CAD build for the part. Positions are in the model's coordinates, mm. Face numbers are marked on the shaded views. A direction names the side the tool comes from. Coordinates: 2 decimals unless noted, no trailing zeros. Loops run counter-clockwise (first coordinate to the right, second up) from the corner with the lowest first, then second, coordinate; pieces in that order, holes last. Notation, with made-up numbers: (-21.75, 6.25) - (19.25, 6.25) arc R11 ccw to (19.25, 16.25) - close; hole circle Ø1 at (-16.75, -28.75). An arc over 180 degrees is marked (long way). Put each result on its own line as item: value.
```python
from build123d import *

# Parameters (mm, degrees)
SCHIZZO1_W                        = 27
SCHIZZO1_H                        = 36
ESTRUSIONE_ESTRUSIONE1_DEPTH      = 4
SCHIZZO10_R                       = 1.75
TAGLIO_ESTRUSIONE5_DEPTH          = 10
SCHIZZO12_W                       = 124
SCHIZZO12_H                       = 2.549259356
ESTRUSIONE_ESTRUSIONE2_DEPTH      = 55
ESTRUSIONE_ESTRUSIONE2_DEPTH_BACK = 55
SCHIZZO14_W                       = 3
SCHIZZO14_H                       = 1.5
ESTRUSIONE_ESTRUSIONE3_DEPTH      = 110
SCHIZZO15_W                       = 27
SCHIZZO15_H                       = 4
TAGLIO_ESTRUSIONE6_DEPTH          = 5
SCHIZZO16_R                       = 13.5
TAGLIO_ESTRUSIONE7_DEPTH          = 10


with BuildPart() as part:
    # Schizzo1 → Estrusione-Estrusione1 (new body)
    with BuildSketch(Plane.XY):
        with Locations((13.5, -18)):
            Rectangle(SCHIZZO1_W, SCHIZZO1_H)
    extrude(amount=ESTRUSIONE_ESTRUSIONE1_DEPTH)

    # Schizzo10 → Taglio-Estrusione5 (cut)
    with BuildSketch(Plane.XY.offset(4)):
        with Locations((3.5, -12.5)):
            Circle(SCHIZZO10_R)
        with Locations((23.5, -12.5)):
            Circle(SCHIZZO10_R)
        with Locations((23.5, -27.5)):
            Circle(SCHIZZO10_R)
        with Locations((3.5, -27.5)):
            Circle(SCHIZZO10_R)
    extrude(amount=-TAGLIO_ESTRUSIONE5_DEPTH, mode=Mode.SUBTRACT)

    # Schizzo12 → Estrusione-Estrusione2 (add, two sides)
    with BuildSketch(Plane(origin=(13.5, 0, 0), x_dir=(0, 0, -1), z_dir=(1, 0, 0))) as estrusione_estrusione2_sk:
        with Locations((-66, -34.725370322)):
            Rectangle(SCHIZZO12_W, SCHIZZO12_H)
    extrude(amount=ESTRUSIONE_ESTRUSIONE2_DEPTH)
    extrude(estrusione_estrusione2_sk.sketch, amount=-ESTRUSIONE_ESTRUSIONE2_DEPTH_BACK)

    # Schizzo14 → Estrusione-Estrusione3 (add)
    with BuildSketch(Plane.ZY.offset(41.5)):
        with Locations((104, -32.700740644)):
            Rectangle(SCHIZZO14_W, SCHIZZO14_H)
        with Locations((119, -32.700740644)):
            Rectangle(SCHIZZO14_W, SCHIZZO14_H)
    extrude(amount=-ESTRUSIONE_ESTRUSIONE3_DEPTH)

    # Schizzo15 → Taglio-Estrusione6 (cut, through all)
    with BuildSketch(Plane.XY.offset(4)):
        with Locations((13.5, -2)):
            Rectangle(SCHIZZO15_W, SCHIZZO15_H)
    extrude(amount=-TAGLIO_ESTRUSIONE6_DEPTH, mode=Mode.SUBTRACT)

    # Schizzo16 → Taglio-Estrusione7 (cut)
    with BuildSketch(Plane(origin=(0, -33.450740644, 0), x_dir=(1, 0, 0), z_dir=(0, 1, 0))):
        with Locations((29.5, -45)):
            Circle(SCHIZZO16_R)
    extrude(amount=-TAGLIO_ESTRUSIONE7_DEPTH, mode=Mode.SUBTRACT)


solid = part.part
```
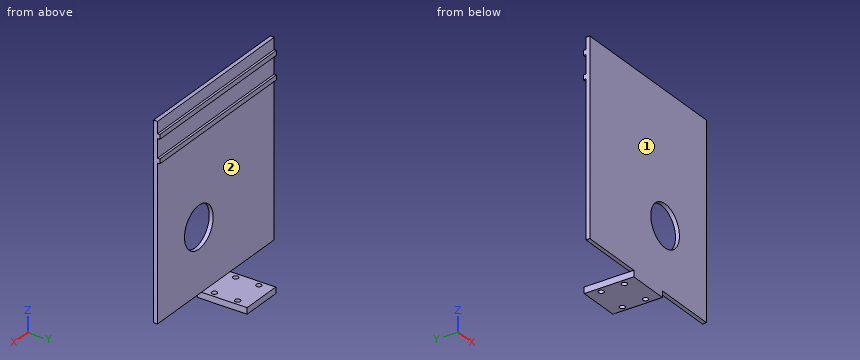
Q1. Slice it at A-A, the plane x = 3.5. Give the cut face in (y, z), then the cut area to 3 significant figures.
Determined:
outline: (-36, 0) - (-29.25, 0) - (-29.25, 4) - (-33.45, 4) - (-33.45, 102.5) - (-31.95, 102.5) - (-31.95, 105.5) - (-33.45, 105.5) - (-33.45, 117.5) - (-31.95, 117.5) - (-31.95, 120.5) - (-33.45, 120.5) - (-33.45, 128) - (-36, 128) - close; (-25.75, 0) - (-14.25, 0) - (-14.25, 4) - (-25.75, 4) - close; (-10.75, 0) - (-4, 0) - (-4, 4) - (-10.75, 4) - close
area: 425 mm2
Q2. Wall check: L1, parallel to Y at x = 23.5, z = 1.2; L2, parallel to X at y = -34.1, z = 45; L3, parallel to Z at x = 29.5, y = -34.95. Give the ranges that are in metal, low to high. Write a range as from..to.
Determined:
L1: -36..-29.25, -25.75..-14.25, -10.75..-4
L2: -41.5..16, 43..68.5
L3: 4..31.5, 58.5..128
Q3. Slice it at D-D, the plane x = 29.5. Give the cut face in (y, z), then the cut area to 3 significant figures.
Determined:
outline: (-36, 4) - (-33.45, 4) - (-33.45, 31.5) - (-36, 31.5) - close; (-36, 58.5) - (-33.45, 58.5) - (-33.45, 102.5) - (-31.95, 102.5) - (-31.95, 105.5) - (-33.45, 105.5) - (-33.45, 117.5) - (-31.95, 117.5) - (-31.95, 120.5) - (-33.45, 120.5) - (-33.45, 128) - (-36, 128) - close
area: 256 mm2
Q4. Pin check, flat tips, straight feed: pin 1 Ø16 at (x, z) = (29.5, 45) entering from -Y; pin 2 Ø5 at (y, z) = (-31, 110.5) entering from +X; pin 3 Ø2 at (x, z) = (-17, 76) entering from +Y; pin 4 Ø2.5 at (x, z) = (-2.5, 119) entering from +Y. Stop position of each tip, or through.
Determined:
pin 1: through
pin 2: x = 68.5
pin 3: y = -33.45
pin 4: y = -31.95
Q5. Tool access for the marked faces 1 and 2: list every direction of +Z, -Z, +X, -X, +Y, -Y with a clear straight run to the whole face (end or side of a thin tool).
Determined:
face 1: +Z, -Z, +X, -X, -Y
face 2: +X, -X, +Y
Q6. Slice it at C-C, the plane y = -12.5. Give the cut face in (x, z).
Determined:
outline: (0, 0) - (1.75, 0) - (1.75, 4) - (0, 4) - close; (5.25, 0) - (21.75, 0) - (21.75, 4) - (5.25, 4) - close; (25.25, 0) - (27, 0) - (27, 4) - (25.25, 4) - close
Q7. Slice it at B-B, the plane z = 45. Give the cut face in (x, y).
Determined:
outline: (-41.5, -36) - (16, -36) - (16, -33.45) - (-41.5, -33.45) - close; (43, -36) - (68.5, -36) - (68.5, -33.45) - (43, -33.45) - close
